For this review, take the finished solid that the model builds, in its own axes (mm). A direction names the side the tool comes from. Coordinates: 2 decimals unless noted, no trailing zeros. Write each loop counter-clockwise with the first axis right and the second up, starting at its lowest first coordinate (ties: lowest second). Pieces come first, ordered by that corner, then holes.
```python
from build123d import *

# Parameters (mm, degrees)
SKETCH1_W                                       = 152.4
SKETCH1_H                                       = 152.4
BOSS_EXTRUDE1_DEPTH                             = 9.525
SKETCH4_W                                       = 63.5
SKETCH4_H                                       = 6.35
CBORE_FOR_10_SOCKET_HEAD_CAP_SCREW1_D           = 5.1054
CBORE_FOR_10_SOCKET_HEAD_CAP_SCREW1_CBORE_D     = 9.525
CBORE_FOR_10_SOCKET_HEAD_CAP_SCREW1_CBORE_DEPTH = 4.826
SKETCH22_R                                      = 47.625
CUT_EXTRUDE3_DEPTH                              = 6.35
SKETCH23_R                                      = 53.2765
SKETCH23_R_2                                    = 50.7365
CUT_EXTRUDE4_DEPTH                              = 1.3462
SKETCH24_R                                      = 17.4625
CUT_EXTRUDE5_DEPTH                              = 25.4
CIRPATTERN1_COUNT                               = 6
SKETCH28_R                                      = 0.635
CUT_EXTRUDE6_DEPTH                              = 10.525
F_6_32_TAPPED_HOLE1_D                           = 2.7051
CIRPATTERN2_COUNT                               = 2
CIRPATTERN2_ANGLE                               = 30
CIRPATTERN3_COUNT                               = 2
CIRPATTERN3_ANGLE                               = 30


with BuildPart() as part:
    # Sketch1 → Boss-Extrude1 (new body)
    with BuildSketch(Plane(origin=(0, 0, 0), x_dir=(-1, 0, 0), z_dir=(0, 0, -1))):
        Rectangle(SKETCH1_W, SKETCH1_H)
    extrude(amount=-BOSS_EXTRUDE1_DEPTH)

    # Sketch4 → Revolve1 (revolve)
    with BuildSketch(Plane(origin=(0, 0, 0), x_dir=(1, 0, 0), z_dir=(0, 1, 0))):
        with Locations((31.75, 3.175)):
            Rectangle(SKETCH4_W, SKETCH4_H)
    revolve(axis=Axis((0, 0, -6.35), (0, 0, 1)))

    # CBORE for #10 Socket Head Cap Screw1 (through all)
    with Locations(Plane(origin=(0, 0, 0), x_dir=(-1, 0, 0), z_dir=(0, 0, -1))):
        with Locations((71.12, 38.1), (71.12, -38.1), (-71.12, 38.1), (-71.12, -38.1), (0, 69.85), (0, -69.85), (71.12, 0), (-71.12, 0)):
            CounterBoreHole(CBORE_FOR_10_SOCKET_HEAD_CAP_SCREW1_D / 2, CBORE_FOR_10_SOCKET_HEAD_CAP_SCREW1_CBORE_D / 2, CBORE_FOR_10_SOCKET_HEAD_CAP_SCREW1_CBORE_DEPTH)

    # Sketch22 → Cut-Extrude3 (cut)
    with BuildSketch(Plane.XY.offset(9.525)):
        Circle(SKETCH22_R)
    extrude(amount=-CUT_EXTRUDE3_DEPTH, mode=Mode.SUBTRACT)

    # Sketch23 → Cut-Extrude4 (cut)
    with BuildSketch(Plane.XY.offset(9.525)):
        Circle(SKETCH23_R)
        Circle(SKETCH23_R_2, mode=Mode.SUBTRACT)
    extrude(amount=-CUT_EXTRUDE4_DEPTH, mode=Mode.SUBTRACT)

    # Sketch24 → Cut-Extrude5 (cut)
    with BuildSketch(Plane.XY.offset(3.175)):
        Circle(SKETCH24_R)
    extrude(amount=-CUT_EXTRUDE5_DEPTH, mode=Mode.SUBTRACT)

    # Sketch25 → #4-40 Tapped Hole1 (revolve, cut)
    with BuildSketch(Plane(origin=(0, 38.1, 3.175), x_dir=(0, -1, 0), z_dir=(1, 0, 0))):
        Polygon((0, 0), (0, 8.273752758), (1.1303, 7.5946), (1.1303, 5.6896), (1.4224, 5.6896), (1.4224, 0), align=None)
    f_4_40_tapped_hole1 = revolve(axis=Axis((0, 38.1, 9.525), (0, 0, -1)), mode=Mode.SUBTRACT)

    # CirPattern1: #4-40 Tapped Hole1 ×6 about axis
    cirpattern1_axis = Axis((0, 0, 0), (0, 0, 1))
    for i in range(1, CIRPATTERN1_COUNT):
        add(f_4_40_tapped_hole1.rotate(cirpattern1_axis, i * 360 / CIRPATTERN1_COUNT), mode=Mode.SUBTRACT)

    # Sketch28 → Cut-Extrude6 (cut, through all)
    with BuildSketch(Plane.XY.offset(3.175)):
        with Locations((0, 28.575)):
            Circle(SKETCH28_R)
    cut_extrude6 = extrude(amount=-CUT_EXTRUDE6_DEPTH, mode=Mode.SUBTRACT)

    # #6-32 Tapped Hole1 (through all)
    with Locations(Plane.XY.offset(3.175)):
        with Locations((0, 28.575)):
            f_6_32_tapped_hole1 = Hole(F_6_32_TAPPED_HOLE1_D / 2)

    # CirPattern2: Cut-Extrude6, #6-32 Tapped Hole1 ×2 about axis
    cirpattern2_axis = Axis((0, 0, 3.175), (0, 0, -1))
    for i in range(1, CIRPATTERN2_COUNT):
        add(cut_extrude6.rotate(cirpattern2_axis, i * CIRPATTERN2_ANGLE / (CIRPATTERN2_COUNT - 1)), mode=Mode.SUBTRACT)
        add(f_6_32_tapped_hole1.rotate(cirpattern2_axis, i * CIRPATTERN2_ANGLE / (CIRPATTERN2_COUNT - 1)), mode=Mode.SUBTRACT)

    # CirPattern3: Cut-Extrude6, #6-32 Tapped Hole1 ×2 about axis
    cirpattern3_axis = Axis((0, 0, 3.175), (0, 0, 1))
    for i in range(1, CIRPATTERN3_COUNT):
        add(cut_extrude6.rotate(cirpattern3_axis, i * CIRPATTERN3_ANGLE / (CIRPATTERN3_COUNT - 1)), mode=Mode.SUBTRACT)
        add(f_6_32_tapped_hole1.rotate(cirpattern3_axis, i * CIRPATTERN3_ANGLE / (CIRPATTERN3_COUNT - 1)), mode=Mode.SUBTRACT)


solid = part.part
```
1) The part is to be moulded in two halves that separate along Y. For faces 4 (the face through (1, 76.2, 5)), 5 (the face through (-0.33, 72.38, 7.21)), 6 (the face through (69.239, -36.375, 7.208)), 7 (the face through (-13, -13, -6.35)), say which applies: pulls with the +Y half, pulls with the -Y half, needs draft (parallel to the pull), parting line crosses it, or undercut.
2) Consider section C-C (x = -10). Give the boundary of the cut face in (y, z) (3 decimals), then the cut area to 3 significant figures.
3) Consider section D-D (x = 41). Give the boundary of the cut face in (y, z) (3 decimals), then the cut area to 3 significant figures.
4) For L1, parallel to Y at x = -71.12, z = 1.5; L2, parallel to Y at x = 71.12, z = 8.5; L3, parallel to Z at x = -59.5, y = 70 (3 decimals), list the stretches that pass through material, from the lowest coordinate up.
5) Clearance check with flat-ended pins moving along their axes: P1, Ø7.5, axis at x = -73, y = 36.5, coming from the -Z side; P2, Ø3, axis at x = 0, y = -38.1, coming from the +Z side (3 decimals); P3, Ø4, axis at x = 54.5, z = -2.5, coming from the -Y side. State where each tip first meets the part, or that it passes through.
6) Consider section B-B (x = -71.12). Give the boundary of the cut face in (y, z) (1 decimal).
7) Tool access review of faces 1 (the face through (28.641, 44.923, 8.861)), 2 (the face through (-69.942, 35.835, 7.208)), 3 (the face through (-73, -2, 4.826)): name each direction out of +Z, -Z, +X, -X, +Y, -Y from which nothing blocks a thin tool from reaching the whole face with its end or side.
8) Consider section A-A (y = -69.85). Give the boundary of the cut face in (x, z) (1 decimal), then the cut area to 3 significant figures.
Results:
1. face 4: pulls with the +Y half
1. face 5: undercut
1. face 6: undercut
1. face 7: needs draft
2. outline: (-76.2, 0) - (-62.708, 0) - (-62.708, -6.35) - (-14.316, -6.35) - (-14.316, 3.175) - (-46.563, 3.175) - (-46.563, 9.525) - (-49.741, 9.525) - (-49.741, 8.179) - (-52.33, 8.179) - (-52.33, 9.525) - (-76.2, 9.525) - close; (14.316, -6.35) - (62.708, -6.35) - (62.708, 0) - (76.2, 0) - (76.2, 9.525) - (52.33, 9.525) - (52.33, 8.179) - (49.741, 8.179) - (49.741, 9.525) - (46.563, 9.525) - (46.563, 3.175) - (14.316, 3.175) - close
2. area: 1,380 mm2
3. outline: (-76.2, 0) - (-48.49, 0) - (-48.49, -6.35) - (48.49, -6.35) - (48.49, 0) - (76.2, 0) - (76.2, 9.525) - (34.02, 9.525) - (34.02, 8.179) - (29.886, 8.179) - (29.886, 9.525) - (24.231, 9.525) - (24.231, 3.175) - (-24.231, 3.175) - (-24.231, 9.525) - (-29.886, 9.525) - (-29.886, 8.179) - (-34.02, 8.179) - (-34.02, 9.525) - (-76.2, 9.525) - close
3. area: 1,750 mm2
4. L1: y = -76.2 to -42.86, -33.34 to -4.76, 4.76 to 33.34, 42.86 to 76.2
4. L2: y = -76.2 to -40.65, -35.55 to -2.55, 2.55 to 35.55, 40.65 to 76.2
4. L3: z = 0 to 9.525
5. P1: stops at z = 0
5. P2: stops at z = 3.175
5. P3: stops at y = -35.72
6. outline: (-76.2, 0) - (-42.9, 0) - (-42.9, 4.8) - (-40.7, 4.8) - (-40.7, 9.5) - (-76.2, 9.5) - close; (-35.5, 4.8) - (-33.3, 4.8) - (-33.3, 0) - (-4.8, 0) - (-4.8, 4.8) - (-2.6, 4.8) - (-2.6, 9.5) - (-35.5, 9.5) - close; (2.6, 4.8) - (4.8, 4.8) - (4.8, 0) - (33.3, 0) - (33.3, 4.8) - (35.5, 4.8) - (35.5, 9.5) - (2.6, 9.5) - close; (40.7, 4.8) - (42.9, 4.8) - (42.9, 0) - (76.2, 0) - (76.2, 9.5) - (40.7, 9.5) - close
7. face 1: +Z
7. face 2: +Z, -Z
7. face 3: -Z
8. outline: (-76.2, 0) - (-4.8, 0) - (-4.8, 4.8) - (-2.6, 4.8) - (-2.6, 9.5) - (-76.2, 9.5) - close; (2.6, 4.8) - (4.8, 4.8) - (4.8, 0) - (76.2, 0) - (76.2, 9.5) - (2.6, 9.5) - close
8. area: 1,380 mm2
